For this review, take the finished solid that the model builds, in its own axes (mm). A direction names the side the tool comes from. Coordinates: 2 decimals unless noted, no trailing zeros. Use one line per item in the form item = value. Start each with the question number.
```python
from build123d import *

# Parameters (mm, degrees)
DODANIE_WYCI_GNI_CIE1_DEPTH = 460
WYTNIJ_WYCI_GNI_CIE1_DEPTH  = 461
SZKIC7_W                    = 5.5
SZKIC7_H                    = 0.01000001
SZKIC8_W                    = 5.5
SZKIC8_H                    = 0.01000001
SZKIC9_W                    = 5.5
SZKIC9_H                    = 0.01000001
SZKIC10_W                   = 5.5
SZKIC10_H                   = 0.01000001
SZKIC11_W                   = 5.5
SZKIC11_H                   = 0.01000001
SZKIC12_W                   = 5.5
SZKIC12_H                   = 0.01000001
SZKIC13_W                   = 5.5
SZKIC13_H                   = 0.01000001
SZKIC14_W                   = 5.5
SZKIC14_H                   = 0.01000001
SFAZOWANIE2_SIZE            = 1.52785882
SFAZOWANIE2_SIZE2           = 1.5207795
SFAZOWANIE4_SIZE            = 1.5207795
SFAZOWANIE4_SIZE2           = 1.52785882
ZAOKR_GLENIE1_R             = 0.499999854
ZAOKR_GLENIE2_R             = 0.999996936


with BuildPart() as part:
    # Szkic1 → Dodanie-wyciągnięcie1 (new body)
    with BuildSketch(Plane.XZ):
        with BuildLine():
            Line((-11.5, 6.269384953), (-11.5, 0))
            Line((-11.5, 0), (11.5, 0))
            Line((11.5, 0), (11.5, 6.269384953))
            Line((11.5, 6.269384953), (7.91556798, 9.879088917))
            Line((7.91556798, 9.879088917), (7.91556798, 13.52061035))
            Line((7.91556798, 13.52061035), (8.93872733, 14.5437697))
            ThreePointArc((8.93872733, 14.5437697), (9.052804678, 14.638756238), (9.13396618, 14.76304982))
            ThreePointArc((9.13396618, 14.76304982), (9.83021824, 15.989534483), (11.095172541, 16.613170738))
            Line((11.095172541, 16.613170738), (11.5, 17.01799817))
            Line((11.5, 17.01799817), (11.5, 18.83162682))
            Line((11.5, 18.83162682), (11.093547074, 19.238079746))
            ThreePointArc((11.093547074, 19.238079746), (9.804732951, 19.879523761), (9.11483221, 21.14306214))
            ThreePointArc((9.11483221, 21.14306214), (9.084093131, 21.201069918), (9.04575086, 21.25435841))
            Line((9.04575086, 21.25435841), (8.30010926, 22.00000001))
            Line((8.30010926, 22.00000001), (-8.30010926, 22.00000001))
            Line((-8.30010926, 22.00000001), (-9.04575086, 21.25435841))
            ThreePointArc((-9.04575086, 21.25435841), (-9.08409312, 21.20106991), (-9.11483221, 21.14306214))
            ThreePointArc((-9.11483221, 21.14306214), (-9.804732946, 19.879523757), (-11.093547072, 19.238079748))
            Line((-11.093547072, 19.238079748), (-11.5, 18.83162682))
            Line((-11.5, 18.83162682), (-11.5, 17.01799817))
            Line((-11.5, 17.01799817), (-11.095172541, 16.613170738))
            ThreePointArc((-11.095172541, 16.613170738), (-9.83021824, 15.989534483), (-9.13396618, 14.76304982))
            ThreePointArc((-9.13396618, 14.76304982), (-9.052804683, 14.638756234), (-8.93872733, 14.5437697))
            Line((-8.93872733, 14.5437697), (-7.91556798, 13.52061035))
            Line((-7.91556798, 13.52061035), (-7.91556798, 9.879088917))
            Line((-7.91556798, 9.879088917), (-11.5, 6.269384953))
        make_face()
    extrude(amount=-DODANIE_WYCI_GNI_CIE1_DEPTH)

    # Szkic2 → Wytnij-wyciągnięcie1 (cut, through all)
    with BuildSketch(Plane(origin=(0, 460, 0), x_dir=(-1, 0, 0), z_dir=(0, 1, 0))):
        Polygon((-2.10671821, 0), (2.10671821, 0), (1.58064429, 0.52607392), (-1.58064429, 0.52607392), align=None)
    extrude(amount=-WYTNIJ_WYCI_GNI_CIE1_DEPTH, mode=Mode.SUBTRACT)

    # Szkic7 → Wycięcie-obrót1 (revolve, cut)
    with BuildSketch(Plane.XZ.offset(-20)):
        with Locations((2.75, 21.995000005)):
            Rectangle(SZKIC7_W, SZKIC7_H)
    revolve(axis=Axis((0, 20, 22.00000001), (0, 0, -1)), mode=Mode.SUBTRACT)

    # Szkic8 → Wycięcie-obrót2 (revolve, cut)
    with BuildSketch(Plane.XZ.offset(-80)):
        with Locations((2.75, 21.995000005)):
            Rectangle(SZKIC8_W, SZKIC8_H)
    revolve(axis=Axis((0, 80, 22.00000001), (0, 0, -1)), mode=Mode.SUBTRACT)

    # Szkic9 → Wycięcie-obrót3 (revolve, cut)
    with BuildSketch(Plane.XZ.offset(-140)):
        with Locations((2.75, 21.995000005)):
            Rectangle(SZKIC9_W, SZKIC9_H)
    revolve(axis=Axis((0, 140, 22.00000001), (0, 0, -1)), mode=Mode.SUBTRACT)

    # Szkic10 → Wycięcie-obrót4 (revolve, cut)
    with BuildSketch(Plane.XZ.offset(-200)):
        with Locations((2.75, 21.995000005)):
            Rectangle(SZKIC10_W, SZKIC10_H)
    revolve(axis=Axis((0, 200, 22.00000001), (0, 0, -1)), mode=Mode.SUBTRACT)

    # Szkic11 → Wycięcie-obrót5 (revolve, cut)
    with BuildSketch(Plane.XZ.offset(-260)):
        with Locations((2.75, 21.995000005)):
            Rectangle(SZKIC11_W, SZKIC11_H)
    revolve(axis=Axis((0, 260, 22.00000001), (0, 0, -1)), mode=Mode.SUBTRACT)

    # Szkic12 → Wycięcie-obrót6 (revolve, cut)
    with BuildSketch(Plane.XZ.offset(-320)):
        with Locations((2.75, 21.995000005)):
            Rectangle(SZKIC12_W, SZKIC12_H)
    revolve(axis=Axis((0, 320, 22.00000001), (0, 0, -1)), mode=Mode.SUBTRACT)

    # Szkic13 → Wycięcie-obrót7 (revolve, cut)
    with BuildSketch(Plane.XZ.offset(-380)):
        with Locations((2.75, 21.995000005)):
            Rectangle(SZKIC13_W, SZKIC13_H)
    revolve(axis=Axis((0, 380, 22.00000001), (0, 0, -1)), mode=Mode.SUBTRACT)

    # Szkic14 → Wycięcie-obrót8 (revolve, cut)
    with BuildSketch(Plane.XZ.offset(-440)):
        with Locations((2.75, 21.995000005)):
            Rectangle(SZKIC14_W, SZKIC14_H)
    revolve(axis=Axis((0, 440, 22.00000001), (0, 0, -1)), mode=Mode.SUBTRACT)

    # Szkic24 → Wycięcie-obrót18 (revolve, cut)
    with BuildSketch(Plane.XZ.offset(-20)):
        Polygon((5.5, 22), (0, 22), (0, 0), (3.5, 0), (3.5, 13), (5.5, 13), align=None)
    revolve(axis=Axis((0, 20, 22), (0, 0, -1)), mode=Mode.SUBTRACT)

    # Szkic25 → Wycięcie-obrót19 (revolve, cut)
    with BuildSketch(Plane.XZ.offset(-80)):
        Polygon((5.5, 22), (0, 22), (0, 0), (3.5, 0), (3.5, 13), (5.5, 13), align=None)
    revolve(axis=Axis((0, 80, 22), (0, 0, -1)), mode=Mode.SUBTRACT)

    # Szkic26 → Wycięcie-obrót20 (revolve, cut)
    with BuildSketch(Plane.XZ.offset(-140)):
        Polygon((5.5, 22), (0, 22), (0, 0), (3.5, 0), (3.5, 13), (5.5, 13), align=None)
    revolve(axis=Axis((0, 140, 22), (0, 0, -1)), mode=Mode.SUBTRACT)

    # Szkic27 → Wycięcie-obrót21 (revolve, cut)
    with BuildSketch(Plane.XZ.offset(-200)):
        Polygon((5.5, 22), (0, 22), (0, 0), (3.5, 0), (3.5, 13), (5.5, 13), align=None)
    revolve(axis=Axis((0, 200, 22), (0, 0, -1)), mode=Mode.SUBTRACT)

    # Szkic28 → Wycięcie-obrót22 (revolve, cut)
    with BuildSketch(Plane.XZ.offset(-260)):
        Polygon((5.5, 22), (0, 22), (0, 0), (3.5, 0), (3.5, 13), (5.5, 13), align=None)
    revolve(axis=Axis((0, 260, 22), (0, 0, -1)), mode=Mode.SUBTRACT)

    # Szkic29 → Wycięcie-obrót23 (revolve, cut)
    with BuildSketch(Plane.XZ.offset(-320)):
        Polygon((5.5, 22), (0, 22), (0, 0), (3.5, 0), (3.5, 13), (5.5, 13), align=None)
    revolve(axis=Axis((0, 320, 22), (0, 0, -1)), mode=Mode.SUBTRACT)

    # Szkic30 → Wycięcie-obrót24 (revolve, cut)
    with BuildSketch(Plane.XZ.offset(-380)):
        Polygon((5.5, 22), (0, 22), (0, 0), (3.5, 0), (3.5, 13), (5.5, 13), align=None)
    revolve(axis=Axis((0, 380, 22), (0, 0, -1)), mode=Mode.SUBTRACT)

    # Szkic31 → Wycięcie-obrót25 (revolve, cut)
    with BuildSketch(Plane.XZ.offset(-440)):
        Polygon((5.5, 22), (0, 22), (0, 0), (3.5, 0), (3.5, 13), (5.5, 13), align=None)
    revolve(axis=Axis((0, 440, 22), (0, 0, -1)), mode=Mode.SUBTRACT)

    # Sfazowanie2
    sfazowanie2_edges = [part.edges().sort_by_distance(p)[0] for p in [
        (11.5, 230, 0),
    ]]
    sfazowanie2_side = [part.faces().sort_by_distance(p)[0] for p in [
        (11.5, 230, 3.134692476),
    ]]
    chamfer(sfazowanie2_edges, length=SFAZOWANIE2_SIZE, length2=SFAZOWANIE2_SIZE2, reference=sfazowanie2_side[0])

    # Sfazowanie4
    sfazowanie4_edges = [part.edges().sort_by_distance(p)[0] for p in [
        (-11.5, 230, 0),
    ]]
    sfazowanie4_side = [part.faces().sort_by_distance(p)[0] for p in [
        (-6.845378829, 230, 0),
    ]]
    chamfer(sfazowanie4_edges, length=SFAZOWANIE4_SIZE, length2=SFAZOWANIE4_SIZE2, reference=sfazowanie4_side[0])

    # Zaokrąglenie1
    zaokr_glenie1_edges = [part.edges().sort_by_distance(p)[0] for p in [
        (-11.095172541, 230, 16.613170738),
        (-11.5, 230, 17.01799817),
        (-11.5, 230, 18.83162682),
        (-11.093547072, 230, 19.238079748),
        (11.093547074, 230, 19.238079746),
        (11.5, 230, 18.83162682),
        (11.5, 230, 17.01799817),
        (11.095172541, 230, 16.613170738),
    ]]
    fillet(zaokr_glenie1_edges, radius=ZAOKR_GLENIE1_R)

    # Zaokrąglenie2
    zaokr_glenie2_edges = [part.edges().sort_by_distance(p)[0] for p in [
        (-7.91556798, 230, 9.879088917),
        (-7.91556798, 230, 13.52061035),
        (7.91556798, 230, 13.52061035),
        (7.91556798, 230, 9.879088917),
        (11.5, 230, 6.269384953),
        (-11.5, 230, 6.269384953),
    ]]
    fillet(zaokr_glenie2_edges, radius=ZAOKR_GLENIE2_R)


solid = part.part
```
1. For pin 1 Ø3.5 at (x, y) = (0.5, 421) entering from -Z; pin 2 Ø1.6 at (x, y) = (0, 179) entering from -Z; pin 3 Ø3.5 at (x, y) = (1, 259.5) entering from +Z; pin 4 Ø4 at (y, z) = (151.5, 8) entering from -X, all flat-tipped, find the tip position at first contact; note any pin that passes through.
2. To check wall thickness, follow line 1 (X direction, y = 79.5, z = 12); line 2 (X direction, y = 320, z = 18.75); line 3 (Z direction, x = -8.5, y = 374.5). State the ranges of each line that lie inside material, in increasing order.
3. The part is to be moulded in two halves that separate along X. For faces 3 (the flat face through (0, 227, 22)), 4 (the cylindrical face through (1.615, 383.105, 6.591)), say which applies: pulls with the +X half, pulls with the -X half, needs draft (parallel to the pull), parting line crosses it, or undercut.
4. Tool access review of faces 1 (the cylindrical face through (-4.05, 16.28, 17.56)), 2 (the cylindrical face through (-0.759, 443.417, 6.591)): name each direction out of +Z, -Z, +X, -X, +Y, -Y from which nothing blocks a thin tool from reaching the whole face with its end or side.
Answers follow:
q1.pin_1 = 0
q1.pin_2 = 0.53
q1.pin_3 = through
q1.pin_4 = -11.49
q2.line_1 = -7.92 to -3.46, 3.46 to 7.92
q2.line_2 = -11.48 to -5.5, 5.5 to 11.48
q2.line_3 = 0 to 9.29, 14.11 to 21.8
q3.face_3 = needs draft
q3.face_4 = undercut
q4.face_1 = +Z
q4.face_2 = +Z, -Z
